```python
from build123d import *

# Parameters (mm, degrees)
HEX_2_DEPTH = 2.5


with BuildPart() as part:
    # BodySke → BaseBody (revolve)
    with BuildSketch(Plane.XY):
        Polygon((0, 0), (0, 1.61), (0.225166605, 2), (7, 2), (8, 1), (7.422649731, 0), align=None)
    revolve(axis=Axis((-12.7, 0, 0), (1, 0, 0)))

    # Sketch2 → Hex 2 (cut)
    with BuildSketch(Plane.ZY):
        Polygon((0.577350269, 1), (-0.577350269, 1), (-1.154700538, 0), (-0.577350269, -1), (0.577350269, -1), (1.154700538, 0), align=None)
    extrude(amount=-HEX_2_DEPTH, mode=Mode.SUBTRACT)


solid = part.part
```
Input: part model. Units: mm. Frame: model coordinates. A direction names the side the tool comes from. Give positions to 0.01 mm unless a question says otherwise; leave off trailing zeros. Write item = value, one per line. Start each with the question number.
1) Reachability of faces 1 (the face through (2.5, 0, 0)), 2 (the face through (7.515, -0.035, -0.156)) from +Z, -Z, +X, -X, +Y, -Y: full face, straight path, thin tool, end or side. Return the list, or none.
2) Material intervals for L1, parallel to Z at x = 1.5, y = 0.75; L2, parallel to Y at x = 1.5, z = 0.7; L3, parallel to X at y = -0.5, z = 1.65, sorted ascending. Write a range as [from, to].
3) Draft query along Z for faces 3 (the face through (1.23, 0.51, -0.86)), 4 (the face through (4, 0, -2)), 5 (the face through (0, 1, 1)). Return one class per face: pulls with the +Z half, pulls with the -Z half, needs draft (parallel to the pull), parting line crosses it, or undercut.
4) Pin query (flat end, axial travel): pin 1 (0.6 mm diameter, centred on y = 0, z = 0, fed in from -X); pin 2 (1.5 mm diameter, centred on x = 3, z = -1.5, fed in from -Y); pin 3 (1 mm diameter, centred on x = 3.5, y = -1, fed in from -Z). Return the tip coordinate at first contact, or that it passes through.
Answers follow:
q1.face_1 = -X
q1.face_2 = +X
q2.L1 = [-1.85, -0.72], [0.72, 1.85]
q2.L2 = [-1.87, -0.79], [0.79, 1.87]
q2.L3 = [0.07, 7.28]
q3.face_3 = undercut
q3.face_4 = parting line crosses it
q3.face_5 = needs draft
q4.pin_1 = 2.5
q4.pin_2 = -1.85
q4.pin_3 = -1.94
